```python
from build123d import *

# Parameters (mm, degrees)
SKETCH1_W           = 34.8
SKETCH1_H           = 34.8
SKETCH1_R           = 13.4
BOSS_EXTRUDE1_DEPTH = 60


with BuildPart() as part:
    # Sketch1 → Boss-Extrude1 (new body)
    with BuildSketch(Plane(origin=(0, 0, 0), x_dir=(1, 0, 0), z_dir=(0, 1, 0))):
        Rectangle(SKETCH1_W, SKETCH1_H)
        with Locations(Location((0, 0, 0), (0, 0, 270))):
            Circle(SKETCH1_R, mode=Mode.SUBTRACT)
    boss_extrude1 = extrude(amount=BOSS_EXTRUDE1_DEPTH)


with BuildPart() as mirror2_1:
    # Mirror2: Boss-Extrude1 across Right Plane
    add(boss_extrude1.mirror(Plane(origin=(0, 0, 0), x_dir=(0, 0, -1), z_dir=(1, 0, 0))))


with BuildPart() as part_1:
    add(part.part)

    # Mirror2 united with what the copies touc: union Mirror2_1
    add(mirror2_1.part)


solid = part_1.part
```
Geometry check sheet. Reference: the model listing, model coordinates, mm. Coordinates: 2 decimals unless noted, no trailing zeros. Order: outer loops, then holes, each group sorted by start corner. A loop starts at its lowest first (then second) coordinate and runs counter-clockwise, first axis right, second up. Notation, with made-up numbers: (19, 88.5) - (62, 88.5) arc R26 ccw to (62, 108.5) - close; hole circle Ø11 at (41.25, 19.25). An arc over 180 degrees is marked (long way). Answer in a Markdown table with one row per item. Add a question column.
1. Draft check along Z on faces 1 (the face through (0, 30, 17.4)), 2 (the face through (-8.2, 29.6, -10.6)), 3 (the face through (7, 0, -12)). Enter one of: +Z half, -Z half, draft (parallel to the pull), parting line (faces both ways), or undercut.
2. Section check C-C (y = 38). Enter the section's corners in (x, z).
3. Section check A-A (z = 0). Enter the section's corners in (x, y), plus the area to 3 significant figures.
4. Section check B-B (x = 0). Enter the section's corners in (y, z).
5. Material ranges on L1, parallel to X at y = 46, z = 0; L2, parallel to X at y = 42, z = 10; L3, parallel to Z at x = 2, y = 43, recorded low to high. Write a range as [from, to].
Data:
| question | item | result |
|---|---|---|
| 1 | face 1 | +Z half |
| 1 | face 2 | undercut |
| 1 | face 3 | draft |
| 2 | outline | (-17.4, -17.4) - (17.4, -17.4) - (17.4, 17.4) - (-17.4, 17.4) - close; hole circle Ø26.8 at (0, 0) |
| 3 | outline | (-17.4, 0) - (-13.4, 0) - (-13.4, 60) - (-17.4, 60) - close; (13.4, 0) - (17.4, 0) - (17.4, 60) - (13.4, 60) - close |
| 3 | area | 480 mm² |
| 4 | outline | (0, -17.4) - (60, -17.4) - (60, -13.4) - (0, -13.4) - close; (0, 13.4) - (60, 13.4) - (60, 17.4) - (0, 17.4) - close |
| 5 | L1 | x = [-17.4, -13.4], [13.4, 17.4] |
| 5 | L2 | x = [-17.4, -8.92], [8.92, 17.4] |
| 5 | L3 | z = [-17.4, -13.25], [13.25, 17.4] |
